from build123d import *

# Parameters (mm, degrees)
SKETCH_2_R                   = 58.5
EXTRUDE_1_DEPTH              = 3
CUT_EXTRUDE_2_DEPTH          = 83.785868359
CUT_EXTRUDE_3_DEPTH          = 83.785868359
SKETCH_5_W                   = 107.181767534
SKETCH_5_H                   = 58.876454488
CUT_EXTRUDE_8_DEPTH          = 83.785868359
FILLET_2_R                   = 5
CUT_EXTRUDE_9_DEPTH          = 83.785868359
FILLET_4_R                   = 5
FILLET_7_R                   = 5
SKETCH_8_W                   = 104
SKETCH_8_H                   = 7.45940389
CUT_EXTRUDE_10_DEPTH         = 0.5
FILLET_8_R                   = 0.5
SKETCH_9_R                   = 2
CUT_EXTRUDE_11_DEPTH         = 10
FILLET_9_R                   = 0.5
HOLE_WIZARD_M3_1_D           = 2.5
HOLE_WIZARD_M3_1_DEPTH       = 3.9
HOLE_WIZARD_M3_1_CSINK_D     = 3.05
HOLE_WIZARD_M3_1_CSINK_ANGLE = 90
HOLE_WIZARD_M3_1_TIP         = 0.751075774


with BuildPart() as part:
    # 草图2 → 凸台-拉伸1 (new body)
    with BuildSketch(Plane(origin=(0, 0, 0), x_dir=(1, 0, 0), z_dir=(0, 1, 0))):
        with Locations(Location((0, 0, 0), (0, 0, 270))):
            Circle(SKETCH_2_R)
    extrude(amount=EXTRUDE_1_DEPTH)

    # 草图3 → 切除-拉伸2 (cut, through all)
    with BuildSketch(Plane.XZ):
        with BuildLine():
            Line((-49.749371855, 5), (49.749371855, 5))
            ThreePointArc((49.749371855, 5), (0, -50), (-49.749371855, 5))
        make_face()
    extrude(amount=-CUT_EXTRUDE_2_DEPTH, mode=Mode.SUBTRACT)

    # 草图4 → 切除-拉伸3 (cut, through all)
    with BuildSketch(Plane(origin=(0, 0, 0), x_dir=(-1, 0, 0), z_dir=(0, -1, 0))):
        with BuildLine():
            Line((-46.56392527, -18.215401819), (46.56392527, -18.215401819))
            ThreePointArc((46.56392527, -18.215401819), (0, -50), (-46.56392527, -18.215401819))
        make_face()
    extrude(amount=-CUT_EXTRUDE_3_DEPTH, mode=Mode.SUBTRACT)

    # 草图5 → 切除-拉伸8 (cut, through all)
    with BuildSketch(Plane(origin=(0, 0, 0), x_dir=(1, 0, 0), z_dir=(0, 1, 0))):
        with Locations((0, -58.5)):
            Rectangle(SKETCH_5_W, SKETCH_5_H)
    extrude(amount=CUT_EXTRUDE_8_DEPTH, mode=Mode.SUBTRACT)

    # 圆角2
    # the kernel refuses this fillet: 5 mm, written as the material it takes off along each edge
    with BuildSketch(Plane(origin=(-50.770693951, 10.80866432, 29.061772756), x_dir=(-0.473436338201062, 0, -0.8808280386492982), z_dir=(0, -1, 0))) as fillet_2_piece_1:
        with BuildLine():
            CenterArc((2.989984287, 4.998217953), FILLET_2_R, 208.257588903, 63.272177489)
            Line((-1.414155907, 2.631036262), (0, 0))
            ThreePointArc((0, 0), (1.561732864, -0.020849951), (3.123465728, 0))
        make_face()
    extrude(amount=18.61732864, mode=Mode.SUBTRACT)
    with BuildSketch(Plane(origin=(50.770693951, 10.80866432, 29.061772756), x_dir=(0.47343633820105957, 0, -0.8808280386492995), z_dir=(0, -1, 0))) as fillet_2_piece_2:
        with BuildLine():
            CenterArc((2.989984287, -4.998217953), FILLET_2_R, 88.470233608, 63.272177489)
            Line((-1.414155907, -2.631036262), (0, 0))
            ThreePointArc((0, 0), (1.561732864, 0.020849951), (3.123465728, 0))
        make_face()
    extrude(amount=18.61732864, mode=Mode.SUBTRACT)
    with BuildSketch(Plane(origin=(-40.686771367, 24.926487598, 29.061772756), x_dir=(-1, 0, 0), z_dir=(0, -1, 0))) as fillet_2_piece_3:
        with BuildLine():
            CenterArc((8.770595039, 5), FILLET_2_R, 154.056362734, 115.943637266)
            ThreePointArc((4.27447082, 7.187433887), (2.287760136, 3.504197713), (0, 0))
            Line((0, 0), (8.770595039, 0))
        make_face()
    extrude(amount=46.852975195, mode=Mode.SUBTRACT)
    with BuildSketch(Plane(origin=(40.686771367, 24.926487598, 29.061772756), x_dir=(1, 0, 0), z_dir=(0, -1, 0))) as fillet_2_piece_4:
        with BuildLine():
            CenterArc((8.770595039, -5), FILLET_2_R, 90, 115.943637266)
            ThreePointArc((4.27447082, -7.187433887), (2.287760136, -3.504197713), (0, 0))
            Line((0, 0), (8.770595039, 0))
        make_face()
    extrude(amount=46.852975195, mode=Mode.SUBTRACT)

    # 草图6 → 切除-拉伸9 (cut, through all)
    with BuildSketch(Plane.XZ):
        with BuildLine():
            Line((-50, 13.34), (-50, 12.34))
            ThreePointArc((-50, 12.34), (-49.707106781, 11.632893219), (-49, 11.34))
            Line((-49, 11.34), (49, 11.34))
            ThreePointArc((49, 11.34), (49.707106781, 11.632893219), (50, 12.34))
            Line((50, 12.34), (50, 13.34))
            ThreePointArc((50, 13.34), (49.707106781, 14.047106781), (49, 14.34))
            Line((49, 14.34), (-49, 14.34))
            ThreePointArc((-49, 14.34), (-49.707106781, 14.047106781), (-50, 13.34))
        make_face()
    extrude(amount=-CUT_EXTRUDE_9_DEPTH, mode=Mode.SUBTRACT)

    # 圆角4
    fillet_4_edges = [part.edges().sort_by_distance(p)[0] for p in [
        (49.749371855, 1.5, 5),
        (-49.749371855, 1.5, 5),
    ]]
    fillet(fillet_4_edges, radius=FILLET_4_R)

    # 圆角7
    fillet_7_edges = [part.edges().sort_by_distance(p)[0] for p in [
        (46.56392527, 1.5, 18.215401819),
        (-46.56392527, 1.5, 18.215401819),
    ]]
    fillet(fillet_7_edges, radius=FILLET_7_R)

    # 草图8 → 切除-拉伸10 (cut)
    with BuildSketch(Plane.XZ):
        with Locations((0, 17.517014665)):
            Rectangle(SKETCH_8_W, SKETCH_8_H)
    extrude(amount=-CUT_EXTRUDE_10_DEPTH, mode=Mode.SUBTRACT)

    # 圆角8
    fillet_8_edges = [part.edges().sort_by_distance(p)[0] for p in [
        (44.089363562, 0.251583272, 21.24671661),
    ]]
    fillet(fillet_8_edges, radius=FILLET_8_R)
    fillet_8_2_edges = [part.edges().sort_by_distance(p)[0] for p in [
        (52, 0.25, 21.24671661),
    ]]
    fillet(fillet_8_2_edges, radius=FILLET_8_R)
    fillet_8_3_edges = [part.edges().sort_by_distance(p)[0] for p in [
        (52, 0.25, 13.78731272),
    ]]
    fillet(fillet_8_3_edges, radius=FILLET_8_R)
    fillet_8_4_edges = [part.edges().sort_by_distance(p)[0] for p in [
        (-52, 0.25, 21.24671661),
    ]]
    fillet(fillet_8_4_edges, radius=FILLET_8_R)
    fillet_8_5_edges = [part.edges().sort_by_distance(p)[0] for p in [
        (-44.089363562, 0.255447628, 21.24671661),
    ]]
    fillet(fillet_8_5_edges, radius=FILLET_8_R)
    # the kernel refuses this fillet: 0.5 mm, written as the material it takes off along each edge
    with BuildSketch(Plane(origin=(49.894377622, 0.5, 13.78731272), x_dir=(0.20668352774517387, 0, -0.9784078491911283), z_dir=(0, -1, 0))) as fillet_8_6_piece_1:
        with BuildLine():
            CenterArc((0.614376094, 0.489203925), FILLET_8_R, 168.071931058, 90)
            Line((0.12517217, 0.592545688), (0.076251777, 0.602879865))
            Line((0.076251777, 0.602879865), (-0.048920392, 0.010334176))
            Line((-0.048920392, 0.010334176), (0.012640058, -0.048375913))
            ThreePointArc((0.012640058, -0.048375913), (0.449150506, -0.0380308), (0.500700154, -0.048920392))
            Line((0.500700154, -0.048920392), (0.51103433, 0))
        make_face()
    extrude(amount=2.014055945, mode=Mode.SUBTRACT)
    # the kernel refuses this fillet: 0.5 mm, written as the material it takes off along each edge
    with BuildSketch(Plane(origin=(-49.894377622, 0.5, 13.78731272), x_dir=(-1, 0, 0), z_dir=(0, -1, 0))) as fillet_8_7_piece_1:
        with BuildLine():
            CenterArc((0.605622378, 0.5), FILLET_8_R, 180, 90)
            Line((0.105622378, 0.5), (0.055622378, 0.5))
            ThreePointArc((0.055622378, 0.5), (0.055622378, 0.44731272), (-0.044718881, 0.022365636))
            Line((-0.044718881, 0.022365636), (0, -0.05))
            Line((0, -0.05), (0.605622378, -0.05))
            Line((0.605622378, -0.05), (0.605622378, 0))
        make_face()
    extrude(amount=2.014055945, mode=Mode.SUBTRACT)

    # 草图9 → 切除-拉伸11 (cut)
    with BuildSketch(Plane(origin=(0, 3, 0), x_dir=(1, 0, 0), z_dir=(0, 1, 0))):
        with Locations((57.07349998, -12.84)):
            Circle(SKETCH_9_R)
        with Locations((-57.07349998, -12.84)):
            Circle(SKETCH_9_R)
    extrude(amount=-CUT_EXTRUDE_11_DEPTH, mode=Mode.SUBTRACT)

    # 圆角9
    fillet_9_edges = [part.edges().sort_by_distance(p)[0] for p in [
        (56.601235389, 1.5, 14.783441832),
        (57.479055827, 1.5, 10.881550497),
        (-57.479055827, 1.5, 10.881550497),
        (-56.601235389, 1.5, 14.783441832),
    ]]
    fillet(fillet_9_edges, radius=FILLET_9_R)

    # M3 螺纹孔1
    with Locations(Plane(origin=(0, 3, 0), x_dir=(1, 0, 0), z_dir=(0, 1, 0))):
        with Locations((53.213363577, 1.475326476), (-53.213363577, 1.668639438), (-0.086594156, 55.526064592), (68.846840655, 52.777963262)):
            CounterSinkHole(HOLE_WIZARD_M3_1_D / 2, HOLE_WIZARD_M3_1_CSINK_D / 2, depth=HOLE_WIZARD_M3_1_DEPTH, counter_sink_angle=HOLE_WIZARD_M3_1_CSINK_ANGLE)
            with Locations((0, 0, -(HOLE_WIZARD_M3_1_DEPTH + HOLE_WIZARD_M3_1_TIP / 2))):  # 118° drill point
                Cone(0, HOLE_WIZARD_M3_1_D / 2, HOLE_WIZARD_M3_1_TIP, mode=Mode.SUBTRACT)


solid = part.part
Build history of the part. All positions in model axes, mm. A direction names the side the tool comes from. Coordinates: 2 decimals unless noted, no trailing zeros. Order: outer loops, then holes, each group sorted by start corner. A loop starts at its lowest first (then second) coordinate and runs counter-clockwise, first axis right, second up. Notation, with made-up numbers: (-30.5, 85) -> (-16.5, 85) arc R21 cw to (-16.5, 121) -> close; hole circle Ø1 at (47, -13.5). An arc over 180 degrees is marked (long way). One line per item, written item: value.
(1) Slice it at A-A, the plane x = 33.5. List the corners of the cut face in (y, z), plus the area to 3 significant figures.
Checked values:
outline: (0, -47.96) -> (3, -47.96) -> (3, -37.12) -> (0, -37.12) -> close; (0, 5) -> (3, 5) -> (3, 11.34) -> (0, 11.34) -> close; (0.5, 14.34) -> (3, 14.34) -> (3, 18.22) -> (0.5, 18.22) -> close
area: 61.2 mm2
(2) Tool access for faces 5 (the flat face through (-1, 1, 5)), 6 (the flat face through (-1, 0.5, 17)), 7 (the cylindrical face through (50.781, 1.521, 28.064)): list every direction of +Z, -Z, +X, -X, +Y, -Y with a clear straight run to the whole face (end or side of a thin tool).
Checked values:
face 5: +Y, -Y
face 6: -Y
face 7: +Z, +X, +Y, -Y
(3) Slice it at B-B, the plane z = -47. List the corners of the cut face in (x, y).
Checked values:
outline: (-34.83, 0) -> (-17.06, 0) -> (-17.06, 3) -> (-34.83, 3) -> close; (17.06, 0) -> (34.83, 0) -> (34.83, 3) -> (17.06, 3) -> close
(4) Mould opens along Z. For faces 1 (the cylindrical face through (-54.406, 1.343, -2.044)), 2 (the cylindrical face through (54.6, 1.5, 21)), 3 (the flat face through (5, 0, 8)), 4 (the cylindrical face through (-55.114, 1.521, 12.438)) say: pulls with the +Z half, pulls with the -Z half, needs draft (parallel to the pull), parting line crosses it, or undercut.
Checked values:
face 1: undercut
face 2: pulls with the +Z half
face 3: needs draft
face 4: undercut
(5) Probe line 1 (X direction, y = 2.5, z = 13); line 2 (Z direction, x = -11, y = 1.5) (1 decimal); line 3 (Z direction, x = -45.5, y = 1.8). List the from-to ranges inside material, lowest first. Write a range as [from, to].
Checked values:
line 1: [-55.08, -50], [50, 55.08]
line 2: [-57.5, -48.8], [5, 11.3], [14.3, 18.2]
line 3: [-36.77, -20.73], [4.97, 11.34], [14.34, 27.12]
(6) Slice it at C-C, the plane x = -19.5. List the corners of the cut face in (y, z), plus the area to 3 significant figures.
Checked values:
outline: (0, -55.15) -> (3, -55.15) -> (3, -46.04) -> (0, -46.04) -> close; (0, 5) -> (3, 5) -> (3, 11.34) -> (0, 11.34) -> close; (0.5, 14.34) -> (3, 14.34) -> (3, 18.22) -> (0.5, 18.22) -> close
area: 56.0 mm2
(7) Drop flat-ended pins along their axis: pin 1 Ø1.1 at (y, z) = (1, 13) entering from -X; pin 2 Ø0.8 at (y, z) = (1.5, 12.5) entering from +X; pin 3 Ø0.6 at (x, y) = (49, 0) entering from -Z; pin 4 Ø1.5 at (x, z) = (-0.09, -55.53) entering from +Y. Give the stop position or say it passes through.
Checked values:
pin 1: x = -55.2
pin 2: x = 55.22
pin 3: z = -32.41
pin 4: through
(8) Slice it at D-D, the plane z = -13. List the corners of the cut face in (x, y).
Checked values:
outline: (-57.04, 0) -> (-48.28, 0) -> (-48.28, 3) -> (-57.04, 3) -> close; (48.28, 0) -> (57.04, 0) -> (57.04, 3) -> (48.28, 3) -> close
